Autodesk Inventor part; units mm, degrees
ref_plane "RisePlane" through (0, 0, 3) normal (0, 0, 1) x (1, 0, 0)
ref_plane "YZ Plane" through (0, 0, 0) normal (1, 0, 0) x (0, 1, 0)
ref_plane "XZ Plane" through (0, 0, 0) normal (0, 1, 0) x (-1, 0, 0)
sketch "Base" plane through (0, 0, 0) normal (0, 0, 1) x (1, 0, 0)
  circle A0 centre (-17.02, -17.02) radius 1.05
  arc A1 (-12.5579, -14.4893) -> (-14.6643, -12.3531) centre (-13.6111, -13.4212) ccw construction
  line L0 (-13.6111, -13.4212) -> (-17.02, -17.02) construction
  circle A2 centre (-13.6111, -13.4212) radius 1.5
  circle A3 centre (-13.6111, -13.4212) radius 3.5
  circle A4 centre (-17.02, -17.02) radius 3.05
  line L1 (-11.2991, -16.0489) -> (-15.0053, -19.3098)
  line L2 (-16.3601, -11.2549) -> (-19.4156, -15.1322)
  point P0 (0, 0)
  point P1 (-15.3155, -15.2206)
  dimension "d3" = 2
  dimension "d4" = 2
extrude "BaseFeature" add sketch "Base" along normal blind 7
ref_plane "RisePlane" through (0, 0, 3) normal (0, 0, 1) x (1, 0, 0)
sketch "RiseProfile" plane through (0, 0, 0) normal (0, 0, -1) x (-1, 0, 0)
  arc A0 (15.0053, -19.3098) -> (19.4156, -15.1322) centre (17.02, -17.02) ccw
  line L0 (16.3601, -11.2549) -> (19.4156, -15.1322)
  circle A1 centre (17.02, -17.02) radius 3.05
  line L1 (15.0053, -19.3098) -> (11.2991, -16.0489)
  arc A2 (16.3601, -11.2549) -> (11.2991, -16.0489) centre (13.6111, -13.4212) ccw
  point P0 (0, 0)
  point P1 (15.0053, -19.3098)
extrude "RiseFeature" cut sketch "RiseProfile" against normal up to surface (3 mm away) contours L1 A2 L0 A1
properties part number "IRLedMount"
Design review of the part built by this model. Coordinates are the model's own, in mm. Coordinates: 2 decimals unless noted, no trailing zeros. Loops run counter-clockwise (first coordinate to the right, second up) from the corner with the lowest first, then second, coordinate; pieces in that order, holes last. Notation, with made-up numbers: M 20.25,-21.75 L 68.25,-21.75 A34 cw 68.25,11.25 Z; hole C 47.25,-29 d7. An arc over 180 degrees is marked long. One line per question, with ' | ' between items.
(1) We need section D-D (y = -18.75). Give the boundary of the cut face in (x, z), and give its area (3 significant figures).
Filled in:
outline: M -19.53,0 L -14.51,0 L -14.51,3 L -14.37,3 L -14.37,7 L -19.53,7 Z | area: 35.7 mm^2
(2) For pin 1 Ø4 at (y, z) = (-18, 1.5) entering from -X; pin 2 Ø2 at (y, z) = (-11, 6) entering from +X, all flat-tipped, find the tip position at first contact; note any pin that passes through.
Filled in:
pin 1: stops at x = -20.07 | pin 2: stops at x = -10.41
(3) We need section C-C (z = 6). Give the boundary of the cut face in (x, y), and give its area (3 significant figures).
Filled in:
outline: M -19.42,-15.13 A3.05 ccw -15.01,-19.31 L -11.3,-16.05 A3.5 ccw long -16.36,-11.25 Z; hole C -17.02,-17.02 d2.1; hole C -13.61,-13.42 d3 | area: 55.9 mm^2
(4) Draft analysis for pull direction X (two halves, no side actions). For faces 1 (the face through (-19.8, -18.27, 2.67)), 2 (the face through (-13, -15, 3)), 3 (the face through (-12.225, -12.847, 4.972)), state which applies: released by +X, released by -X, zero draft, split by the parting line, or undercut.
Filled in:
face 1: split by the parting line | face 2: zero draft | face 3: undercut
(5) Wall thickness on probe 1 along Z at (x, y) = (-11.5, -15); probe 2 along X at (y, z) = (-14, 5.5); probe 3 along X at (y, z) = (-12.5, 6.25): over which ranges is each line inside the solid? List them lowest first.
Filled in:
probe 1: z = 3 to 7 | probe 2: x = -18.52 to -14.99, -12.23 to -10.16 | probe 3: x = -17.34 to -14.79, -12.43 to -10.23
(6) We need section B-B (y = -16.5). Give the boundary of the cut face in (x, z), and give its area (3 significant figures).
Filled in:
outline: M -20.03,0 L -17.93,0 L -17.93,7 L -20.03,7 Z; M -16.11,0 L -14.01,0 L -14.01,3 L -11.81,3 L -11.81,7 L -16.11,7 Z | area: 38.1 mm^2
(7) We need section A-A (x = -16.5). Give the boundary of the cut face in (y, z).
Filled in:
outline: M -20.03,0 L -17.93,0 L -17.93,7 L -20.03,7 Z; M -16.11,0 L -14.01,0 L -14.01,3 L -11.43,3 L -11.43,7 L -16.11,7 Z
